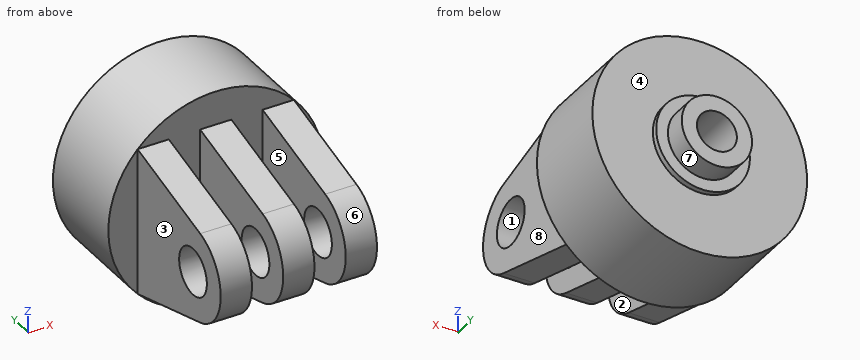
```python
from build123d import *

# Parameters (mm, degrees)
F0_R      = 3.175
F1_DEPTH  = 10.5833333333
F2_R      = 14.544643177
F3_DEPTH  = 12.7
F4_W      = 4.2333333333
F4_H      = 19.05
F5_DEPTH  = 76.2
F6_R      = 6.35
F7_DEPTH  = 0.762
F8_R      = 4.7625
F9_DEPTH  = 3.175
F11_D     = 5.4102
F11_DEPTH = 13.97
F11_TIP   = 1.6253880605


with BuildPart() as f1:
    # F0 (on Right) → F1 (new body, symmetric)
    with BuildSketch(Plane.YZ):
        with BuildLine():
            ThreePointArc((-14.3435009364, 6.1336289969), (-19.05, 0), (-14.3435009364, -6.1336289969))
            Line((-14.3435009364, -6.1336289969), (0, -9.9769584895))
            Line((0, -9.9769584895), (0, 9.9769584895))
            Line((0, 9.9769584895), (-14.3435009364, 6.1336289969))
        make_face()
        with Locations((-12.7, 0)):
            Circle(F0_R, mode=Mode.SUBTRACT)
    extrude(amount=F1_DEPTH, both=True)

    # F2 (on Front) → F3 (join)
    with BuildSketch(Plane.XZ):
        Circle(F2_R)
    extrude(amount=-F3_DEPTH)

    # F4 (on Top) → F5 (cut, symmetric)
    with BuildSketch(Plane.XY):
        with Locations((-4.2333333333, -9.525)):
            Rectangle(F4_W, F4_H)
        with Locations((4.2333333333, -9.525)):
            Rectangle(F4_W, F4_H)
    extrude(amount=F5_DEPTH, both=True, mode=Mode.SUBTRACT)

    # F6 (on face) → F7 (join)
    with BuildSketch(Plane(origin=(0, 12.7, 0), x_dir=(-1, 0, 0), z_dir=(0, 1, 0))):
        Circle(F6_R)
    extrude(amount=F7_DEPTH)

    # F8 (on face) → F9 (join)
    with BuildSketch(Plane(origin=(0, 13.462, 0), x_dir=(-1, 0, 0), z_dir=(0, 1, 0))):
        Circle(F8_R)
    extrude(amount=F9_DEPTH)

    # F11
    with Locations(Plane(origin=(0, 16.637, 0), x_dir=(-1, 0, 0), z_dir=(0, 1, 0))):
        with Locations((0, 0)):
            Hole(F11_D / 2, depth=F11_DEPTH)
            with Locations((0, 0, -(F11_DEPTH + F11_TIP / 2))):  # 118° drill point
                Cone(0, F11_D / 2, F11_TIP, mode=Mode.SUBTRACT)


solid = f1.part
```
The model under review builds one solid part; all positions refer to its coordinate system, in mm. Face numbers are marked on the shaded views. A direction names the side the tool comes from. Round coordinates to 2 decimals unless told otherwise and drop trailing zeros. Loops run counter-clockwise (first coordinate to the right, second up) from the corner with the lowest first, then second, coordinate; pieces in that order, holes last.
1) Consider section C-C on z = -5.5. State the section outline as (x, y) points.
Values follow:
outline: (-13.46, 0) - (-10.58, 0) - (-10.58, -15.87) - (-6.35, -15.87) - (-6.35, 0) - (-2.12, 0) - (-2.12, -15.87) - (2.12, -15.87) - (2.12, 0) - (6.35, 0) - (6.35, -15.87) - (10.58, -15.87) - (10.58, 0) - (13.46, 0) - (13.46, 12.7) - (3.17, 12.7) - (3.17, 13.46) - (-3.17, 13.46) - (-3.17, 12.7) - (-13.46, 12.7) - close
2) Clearance check with flat-ended pins moving along their axes: P1, Ø2, axis at x = -8, z = -7.5, coming from the +Y side; P2, Ø3, axis at x = -11.5, y = 11.5, coming from the +Z side; P3, Ø10, axis at y = -13, z = 8.5, coming from the -X side. State where each tip first meets the part, or that it passes through.
Values follow:
P1: stops at y = 12.7
P2: stops at z = 10.56
P3: stops at x = -10.58
3) Wall thickness on line 1 along X through (y, z) = (-7.5, -7.75); line 2 along X through (y, z) = (5.75, 0): over which ranges is each line inside the solid? List them lowest first.
Values follow:
line 1: x = -10.58 to -6.35, -2.12 to 2.12, 6.35 to 10.58
line 2: x = -14.54 to -2.71, 2.71 to 14.54
4) Consider section A-A on y = -12.7. State the section outline as (x, z) points (3 decimals).
Values follow:
outline: (-10.583, -6.574) - (-6.35, -6.574) - (-6.35, -3.175) - (-10.583, -3.175) - close; (-10.583, 3.175) - (-6.35, 3.175) - (-6.35, 6.574) - (-10.583, 6.574) - close; (-2.117, -6.574) - (2.117, -6.574) - (2.117, -3.175) - (-2.117, -3.175) - close; (-2.117, 3.175) - (2.117, 3.175) - (2.117, 6.574) - (-2.117, 6.574) - close; (6.35, -6.574) - (10.583, -6.574) - (10.583, -3.175) - (6.35, -3.175) - close; (6.35, 3.175) - (10.583, 3.175) - (10.583, 6.574) - (6.35, 6.574) - close
5) Consider section D-D on y = 6.5. State the section outline as (x, z) points, then the cut area to 3 significant figures.
Values follow:
outline: circle Ø29.09 at (0, 0); hole circle Ø5.41 at (0, 0)
area: 642 mm2
6) The part is to be moulded in two halves that separate along X. For the marked faces 5, 6, 7 and 8, say which applies: pulls with the +X half, pulls with the -X half, needs draft (parallel to the pull), parting line crosses it, or undercut.
Values follow:
face 5: undercut
face 6: needs draft
face 7: parting line crosses it
face 8: pulls with the +X half
7) Tool access review of the marked faces 1, 2, 3 and 4: name each direction out of +Z, -Z, +X, -X, +Y, -Y from which nothing blocks a thin tool from reaching the whole face with its end or side.
Values follow:
face 1: +X, -X
face 2: +Z, -Z, -Y
face 3: +Z, -Z, -X, -Y
face 4: +Y
